from build123d import *

# Parameters (mm, degrees)
SKETCH1_W           = 5
SKETCH1_H           = 12.25
BOSS_EXTRUDE1_DEPTH = 5.6
SKETCH3_W           = 2.5
SKETCH3_H           = 3.5
SKETCH3_W_2         = 1
SKETCH3_H_2         = 0.4
BOSS_EXTRUDE2_DEPTH = 3
SKETCH4_W           = 5.6
SKETCH4_H           = 0.75
BOSS_EXTRUDE3_DEPTH = 2.25
SKETCH5_W           = 2.25
SKETCH5_H           = 0.75
BOSS_EXTRUDE4_DEPTH = 10.75


with BuildPart() as part:
    # Sketch1 → Boss-Extrude1 (new body)
    with BuildSketch(Plane.XY):
        with Locations((2.5, 6.125)):
            Rectangle(SKETCH1_W, SKETCH1_H)
    extrude(amount=BOSS_EXTRUDE1_DEPTH)

    # Sketch3 → Boss-Extrude2 (add)
    with BuildSketch(Plane(origin=(5, 0, 0), x_dir=(0, 0, -1), z_dir=(1, 0, 0))):
        with Locations((-2.85, 6.125)):
            Rectangle(SKETCH3_W, SKETCH3_H)
        with Locations((-2.6, 6.625)):
            Rectangle(SKETCH3_W_2, SKETCH3_H_2, mode=Mode.SUBTRACT)
        with Locations((-2.6, 5.625)):
            Rectangle(SKETCH3_W_2, SKETCH3_H_2, mode=Mode.SUBTRACT)
    extrude(amount=BOSS_EXTRUDE2_DEPTH)

    # Sketch4 → Boss-Extrude3 (add)
    with BuildSketch(Plane.ZY):
        with Locations((2.8, 11.875)):
            Rectangle(SKETCH4_W, SKETCH4_H)
        with Locations((2.8, 0.375)):
            Rectangle(SKETCH4_W, SKETCH4_H)
    extrude(amount=BOSS_EXTRUDE3_DEPTH)

    # Sketch5 → Boss-Extrude4 (add)
    with BuildSketch(Plane.XZ.offset(-11.5)):
        with Locations((-1.125, 5.225)):
            Rectangle(SKETCH5_W, SKETCH5_H)
    extrude(amount=BOSS_EXTRUDE4_DEPTH)


solid = part.part
Read the model definition and answer for the solid it produces. Units are mm, in the model's axes. A direction names the side the tool comes from. Give positions to 0.01 mm unless a question says otherwise; leave off trailing zeros. Write each loop counter-clockwise with the first axis right and the second up, starting at its lowest first coordinate (ties: lowest second). Pieces come first, ordered by that corner, then holes. Notation, with made-up numbers: (82.25, -1) - (112.25, -1) arc R19 cw to (112.25, 35) - close; hole circle Ø8 at (37, 47). An arc over 180 degrees is marked (long way). Use CSV: the item, a comma, the result in double quotes. Start each with the question number.
Item 1: The part is cut by section D-D, the plane z = 3.8. Give the vertices of the cut face in (x, y) (3 decimals), and give its area (3 significant figures).
Item 2: The mould has two halves that part along Y. Classify faces 1 (the flat face through (8, 6, 3)), 2 (the flat face through (1, 12.25, 3)), 3 (the flat face through (6.5, 6.825, 2.6)): pulls with the +Y half, pulls with the -Y half, needs draft (parallel to the pull), parting line crosses it, or undercut.
Item 3: The part is cut by section A-A, the plane z = 0.5. Give the vertices of the cut face in (x, y).
Item 4: Consider line 1 (Z direction, x = 7, y = 5.5); line 2 (Y direction, x = -1, z = 0.4); line 3 (X direction, y = 11.25, z = 0.55). Determine where each line is inside the solid, lowest interval first.
Item 5: For faces 4 (the flat face through (6, 6, 1.6)), 5 (the flat face through (6, 6, 4.1)), 6 (the flat face through (6.5, 5.825, 2.6)), 7 (the flat face through (-1, 0.75, 2)), 8 (the flat face through (6, 7.875, 3)), determine the directions among +Z, -Z, +X, -X, +Y, -Y from which every point of the face is accessible in a straight line to the end or side of a thin tool.
Item 6: The part is cut by section C-C, the plane y = 10. Give the vertices of the cut face in (x, z).
Item 7: The part is cut by section B-B, the plane x = 7. Give the vertices of the cut face in (y, z) (3 decimals), and give its area (3 significant figures).
Item 8: Flat-ended cylindrical pins translate along their axes: P1, Ø1.8, axis at x = -1.5, y = 5, coming from the -Z side; P2, Ø1.1, axis at x = 6.5, z = 2.5, coming from the +Y side (3 decimals); P3, Ø2, axis at y = 11, z = 1.5, coming from the +X side. Find the tip coordinate at first contact, or state that the pin passes through.
Taken from the geometry:
1,outline,"(-2.25, 0) - (5, 0) - (5, 4.375) - (8, 4.375) - (8, 7.875) - (5, 7.875) - (5, 12.25) - (-2.25, 12.25) - (-2.25, 11.5) - (0, 11.5) - (0, 0.75) - (-2.25, 0.75) - close"
1,area,"75.1 mm2"
2,face 1,"needs draft"
2,face 2,"pulls with the +Y half"
2,face 3,"undercut"
3,outline,"(-2.25, 0) - (5, 0) - (5, 12.25) - (-2.25, 12.25) - (-2.25, 11.5) - (0, 11.5) - (0, 0.75) - (-2.25, 0.75) - close"
4,line 1,"1.6 to 2.1, 3.1 to 4.1"
4,line 2,"0 to 0.75, 11.5 to 12.25"
4,line 3,"0 to 5"
5,face 4,"-Z, +X, +Y, -Y"
5,face 5,"+Z, +X, +Y, -Y"
5,face 6,"+X"
5,face 7,"-Z, -X"
5,face 8,"+Z, -Z, +X, +Y"
6,outline,"(-2.25, 4.85) - (0, 4.85) - (0, 0) - (5, 0) - (5, 5.6) - (-2.25, 5.6) - close"
7,outline,"(4.375, 1.6) - (7.875, 1.6) - (7.875, 4.1) - (4.375, 4.1) - close; hole (5.425, 2.1) - (5.825, 2.1) - (5.825, 3.1) - (5.425, 3.1) - close; hole (6.425, 2.1) - (6.825, 2.1) - (6.825, 3.1) - (6.425, 3.1) - close"
7,area,"7.95 mm2"
8,P1,"z = 4.85"
8,P2,"y = 7.875"
8,P3,"x = 5"
